from build123d import *

# Parameters (mm, degrees)
SKETCH1_R           = 3.96875
SKETCH1_R_2         = 2
BOSS_EXTRUDE1_DEPTH = 8.89


with BuildPart() as part:
    # Sketch1 → Boss-Extrude1 (new body)
    with BuildSketch(Plane(origin=(0, 0, 0), x_dir=(1, 0, 0), z_dir=(0, 1, 0))):
        with BuildLine():
            Line((80.3275, 31.75), (-7.9375, 31.75))
            Line((-7.9375, 31.75), (-7.9375, 13.97))
            Line((-7.9375, 13.97), (-7.9375, 0))
            ThreePointArc((-7.9375, 0), (0, -7.9375), (7.9375, 0))
            Line((7.9375, 0), (27.888727654, 13.97))
            Line((27.888727654, 13.97), (44.501272346, 13.97))
            Line((44.501272346, 13.97), (64.4525, 0))
            ThreePointArc((64.4525, 0), (72.39, -7.9375), (80.3275, 0))
            Line((80.3275, 0), (80.3275, 13.97))
            Line((80.3275, 13.97), (80.3275, 31.75))
        make_face()
        with Locations(Location((0, 0, 0), (0, 0, 270))):
            Circle(SKETCH1_R, mode=Mode.SUBTRACT)
        with Locations(Location((72.39, 0, 0), (0, 0, 270))):
            Circle(SKETCH1_R, mode=Mode.SUBTRACT)
        with Locations(Location((72.39, 22.86, 0), (0, 0, 270))):
            Circle(SKETCH1_R, mode=Mode.SUBTRACT)
        with Locations(Location((0, 22.86, 0), (0, 0, 270))):
            Circle(SKETCH1_R, mode=Mode.SUBTRACT)
        with Locations(Location((11.43, 8.89, 0), (0, 0, 270))):
            Circle(SKETCH1_R_2, mode=Mode.SUBTRACT)
    extrude(amount=-BOSS_EXTRUDE1_DEPTH)


solid = part.part
Check sheet for the modelled part. Datum: model origin and axes. Units: mm. A direction names the side the tool comes from. Round coordinates to 2 decimals unless told otherwise and drop trailing zeros. Loops run counter-clockwise (first coordinate to the right, second up) from the corner with the lowest first, then second, coordinate; pieces in that order, holes last. Notation, with made-up numbers: (43, -34.5) - (78, -34.5) arc R13 ccw to (78, -28.5) - close; hole circle Ø4 at (18.5, 75). An arc over 180 degrees is marked (long way). Answer as CSV lines item,"result". Start each with the question number.
Item 1: Section check D-D (x = 43). Record the boundary of the cut face in (y, z), and give its area (3 significant figures).
Item 2: Scan lines: line 1 (X direction, y = -2.25, z = -22.86); line 2 (X direction, y = -7.25, z = -21.5); line 3 (X direction, y = -2.5, z = -3). Record each from-to range of solid material in increasing order. Write a range as [from, to].
Item 3: Section check A-A (x = 72.39). Record the boundary of the cut face in (y, z).
Item 4: Depth check by flat-ended pin: P1, Ø4.5, axis at x = 33.5, y = -3, coming from the +Z side; P2, Ø6.5, axis at x = 11.43, z = -8.89, coming from the -Y side. Enter the tip coordinate at first touch or a pass-through.
Item 5: Release check for a two-part mould opening along X. For faces 1 (the cylindrical face through (-0.175, -4.383, 7.936)), 2 (the flat face through (36, -8.89, -17)), 3 (the flat face through (-7.938, -4, -16)), 4 (the flat face through (17.773, -4.383, -6.887)) record: +X half, -X half, draft (parallel to the pull), parting line (faces both ways), or undercut.
Item 6: Set-up check for faces 5 (the flat face through (54.34, -4.38, -7.08)), 6 (the cylindrical face through (68.516, -4.383, -23.72)): record each of +Z, -Z, +X, -X, +Y, -Y from which the full face is reachable in a straight line by a thin tool's end or side.
Item 7: Section check B-B (y = -7). Count the separate pieces of the cut face and the enclosed holes in it, and give its area (3 significant figures).
Item 8: Section check C-C (z = -23). Record the boundary of the cut face in (x, y), and give its area (3 significant figures).
Report:
1,outline,"(-8.89, -31.75) - (0, -31.75) - (0, -13.97) - (-8.89, -13.97) - close"
1,area,"158 mm2"
2,line 1,"x = [-7.94, -3.97], [3.97, 68.42], [76.36, 80.33]"
2,line 2,"x = [-7.94, -3.73], [3.73, 68.66], [76.12, 80.33]"
2,line 3,"x = [-7.94, -2.6], [2.6, 12.22], [60.17, 69.79], [74.99, 80.33]"
3,outline,"(-8.89, -31.75) - (0, -31.75) - (0, -26.83) - (-8.89, -26.83) - close; (-8.89, -18.89) - (0, -18.89) - (0, -3.97) - (-8.89, -3.97) - close; (-8.89, 3.97) - (0, 3.97) - (0, 7.94) - (-8.89, 7.94) - close"
4,P1,"stops at z = -13.97"
4,P2,"stops at y = -8.89"
5,face 1,"undercut"
5,face 2,"draft"
5,face 3,"-X half"
5,face 4,"undercut"
6,face 5,"+Z, +Y, -Y"
6,face 6,"+Y, -Y"
7,separate pieces,"1"
7,enclosed holes,"5"
7,area,"2,280 mm2"
8,outline,"(-7.94, -8.89) - (-3.97, -8.89) - (-3.97, 0) - (-7.94, 0) - close; (3.97, -8.89) - (68.42, -8.89) - (68.42, 0) - (3.97, 0) - close; (76.36, -8.89) - (80.33, -8.89) - (80.33, 0) - (76.36, 0) - close"
8,area,"644 mm2"
